The drawing under review shows one solid part. Ordinate dimensions are in mm from its lowest x, y, z. A direction names the side the tool comes from. Give positions to 0.01 mm unless a question says otherwise; leave off trailing zeros. Loops run counter-clockwise (first coordinate to the right, second up) from the corner with the lowest first, then second, coordinate; pieces in that order, holes last. Notation, with made-up numbers: M 78.5,67.5 L 123.5,67.5 A19 ccw 123.5,74.5 Z; hole C -31.5,30.5 d3. An arc over 180 degrees is marked long. Write item = value, one per line. Start each with the question number.
1. Draft analysis for pull direction Z (two halves, no side actions). For the marked faces 1, 2, 3 and 4, state which applies: pulls with the +Z half, pulls with the -Z half, needs draft (parallel to the pull), parting line crosses it, or undercut.
2. We need section D-D on y = 21.25. Give the boundary of the cut face in (x, z).
3. We need section C-C on x = 17.5. Give the boundary of the cut face in (y, z), then the cut area to 3 significant figures.
4. We need section B-B on z = 2.25. Count the separate pieces of the cut face and the enclosed holes in it, then the cut area to 3 significant figures.
5. Wall thickness on line 1 along Y through (x, z) = (8.25, 1.5) (1 decimal); line 2 along Z through (x, y) = (19.25, 1.5); line 3 along Y through (x, z) = (3, 3.75): over which ranges is each line inside the solid? List them lowest first. Write a range as from..to.
6. For the marked faces 5, 6 and 7, list the 3-axis set-ups (+Z, -Z, +X, -X, +Y, -Y) from which the entire face can be reached by the end or side of a thin tool; tool diameter is ignored.
7. We need section A-A on y = 11. Give the boundary of the cut face in (x, z), then the cut area to 3 significant figures.
8. For pin 1 (3.5 mm diameter, centred on x = 25.654, z = 12.827, fed in from -Y); pin 2 (8.5 mm diameter, centred on x = 8, z = 10.5, fed in from -Y); pin 3 (1 mm diameter, centred on x = 4, z = 2.5, fed in from +Y), all flat-tipped, find the tip position at first contact; note any pin that passes through.
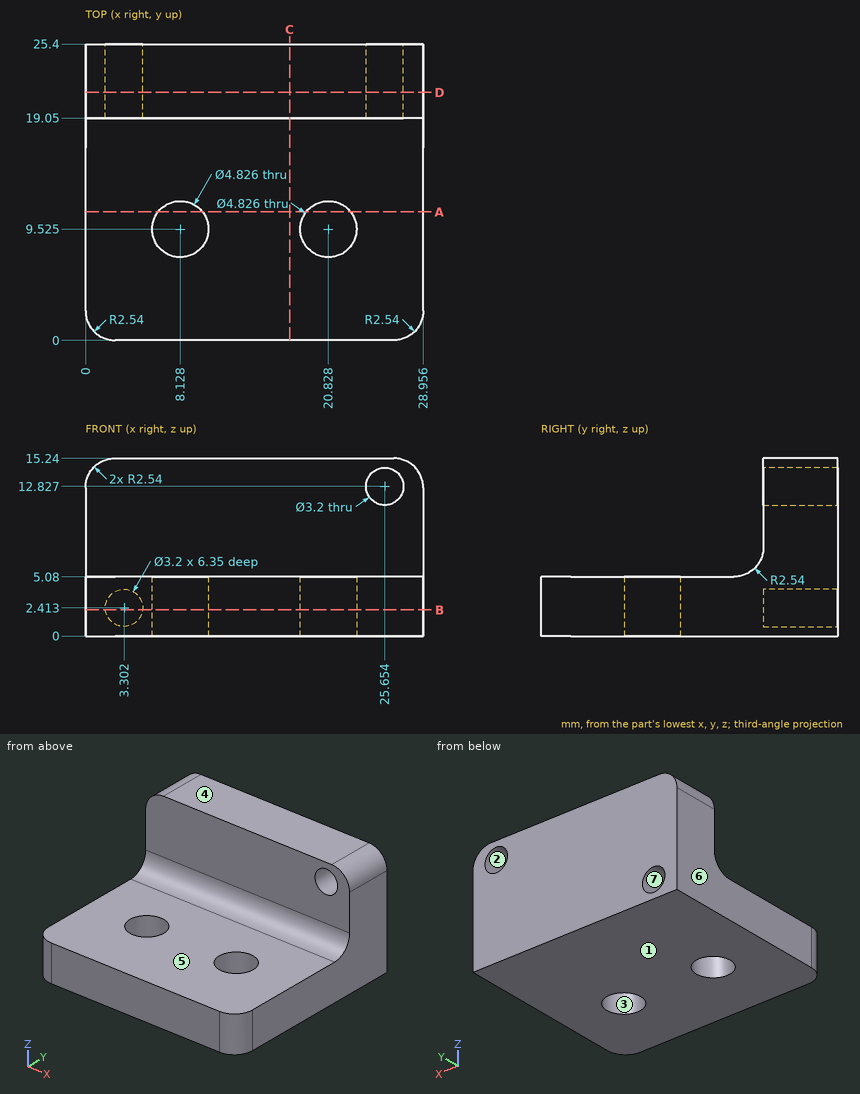
Final values:
q1.face_1 = pulls with the -Z half
q1.face_2 = undercut
q1.face_3 = needs draft
q1.face_4 = pulls with the +Z half
q2.outline = M 0,0 L 28.96,0 L 28.96,12.7 A2.54 ccw 26.42,15.24 L 2.54,15.24 A2.54 ccw 0,12.7 Z; hole C 3.3,2.41 d3.2; hole C 25.65,12.83 d3.2
q3.outline = M 0,0 L 25.4,0 L 25.4,15.24 L 19.05,15.24 L 19.05,7.62 A2.54 cw 16.51,5.08 L 0,5.08 Z
q3.area = 195 mm²
q4.separate_pieces = 1
q4.enclosed_holes = 2
q4.area = 676 mm²
q5.line_1 = 0..7.1, 11.9..25.4
q5.line_2 = 0..5.08
q5.line_3 = 0..19.05
q6.face_5 = +Z, +X, -X, -Y
q6.face_6 = +Z, -Z, -X, +Y, -Y
q6.face_7 = +Y
q7.outline = M 0,0 L 6.22,0 L 6.22,5.08 L 0,5.08 Z; M 10.04,0 L 18.92,0 L 18.92,5.08 L 10.04,5.08 Z; M 22.74,0 L 28.96,0 L 28.96,5.08 L 22.74,5.08 Z
q7.area = 108 mm²
q8.pin_1 = 19.05
q8.pin_2 = 18.65
q8.pin_3 = 19.05
